Geometry check sheet. Reference: the model listing, model coordinates, mm. Face numbers are marked on the shaded views. A direction names the side the tool comes from. Round coordinates to 2 decimals unless told otherwise and drop trailing zeros. Loops run counter-clockwise (first coordinate to the right, second up) from the corner with the lowest first, then second, coordinate; pieces in that order, holes last. Notation, with made-up numbers: M 50,52 L 56,52 A20 cw 56,87 Z; hole C -35.75,31 d8. An arc over 180 degrees is marked long. Answer in a Markdown table with one row per item. Add a question column.
```python
from build123d import *

# Parameters (mm, degrees)
SKETCH1_W             = 150
SKETCH1_H             = 300
BOSS_EXTRUDE1_DEPTH   = 40
SKETCH2_R             = 25
BOSS_EXTRUDE2_DEPTH   = 5
SKETCH3_W             = 40
SKETCH3_H             = 120
CUT_EXTRUDE1_DEPTH    = 5
CUT_EXTRUDE2_DEPTH    = 5
CHAMFER2_SIZE         = 10
CHAMFER3_SIZE         = 2
CHAMFER4_SIZE         = 1
CHAMFER5_SIZE         = 1
CHAMFER6_SIZE         = 6
BODY_MOVE_COPY1_ANGLE = 120


with BuildPart() as part:
    # Sketch1 → Boss-Extrude1 (new, symmetric)
    with BuildSketch(Plane(origin=(0, 0, 0), x_dir=(1, 0, 0), z_dir=(0, 1, 0))):
        Rectangle(SKETCH1_W, SKETCH1_H)
    extrude(amount=BOSS_EXTRUDE1_DEPTH, both=True)

    # Sketch2 → Boss-Extrude2 (add)
    with BuildSketch(Plane.XY.offset(150)):
        with Locations(Location((-40, 0, 0), (0, 0, 180))):
            Circle(SKETCH2_R)
        with Locations(Location((40, 0, 0), (0, 0, 180))):
            Circle(SKETCH2_R)
    boss_extrude2 = extrude(amount=BOSS_EXTRUDE2_DEPTH)

    # Sketch3 → Cut-Extrude1 (cut)
    with BuildSketch(Plane(origin=(0, 40, 0), x_dir=(1, 0, 0), z_dir=(0, 1, 0))):
        Rectangle(SKETCH3_W, SKETCH3_H)
    extrude(amount=-CUT_EXTRUDE1_DEPTH, mode=Mode.SUBTRACT)

    # Sketch4 → Cut-Extrude2 (cut)
    with BuildSketch(Plane(origin=(0, 40, 0), x_dir=(1, 0, 0), z_dir=(0, 1, 0))):
        Polygon((0, -130), (-45, -90), (-26.937608132, -90), (0, -113.944540562), (26.937608132, -90), (45, -90), align=None)
    extrude(amount=-CUT_EXTRUDE2_DEPTH, mode=Mode.SUBTRACT)

    # Chamfer2
    chamfer2_edges = [part.edges().sort_by_distance(p)[0] for p in [
        (75, 40, 0),
        (-75, 40, 0),
        (75, -40, 0),
        (-75, -40, 0),
    ]]
    chamfer(chamfer2_edges, length=CHAMFER2_SIZE)

    # Chamfer3
    chamfer3_edges = [part.edges().sort_by_distance(p)[0] for p in [
        (-20, 35, 0),
        (0, 35, -60),
        (20, 35, 0),
        (0, 35, 60),
        (-20, 40, 0),
        (0, 40, 60),
        (20, 40, 0),
        (0, 40, -60),
        (22.5, 35, 110),
        (-22.5, 35, 110),
        (-35.968804066, 35, 90),
        (-13.468804066, 35, 101.972270281),
        (13.468804066, 35, 101.972270281),
        (35.968804066, 35, 90),
        (22.5, 40, 110),
        (35.968804066, 40, 90),
        (13.468804066, 40, 101.972270281),
        (-13.468804066, 40, 101.972270281),
        (-35.968804066, 40, 90),
        (-22.5, 40, 110),
    ]]
    chamfer(chamfer3_edges, length=CHAMFER3_SIZE)

    # Mirror1: Boss-Extrude2 across plane
    add(boss_extrude2.mirror(Plane.XY))

    # Chamfer4
    chamfer4_edges = [part.edges().sort_by_distance(p)[0] for p in [
        (-15, 0, -155),
        (65, 0, -155),
        (-15, 0, 155),
        (65, 0, 155),
    ]]
    chamfer(chamfer4_edges, length=CHAMFER4_SIZE)

    # Chamfer5
    chamfer5_edges = [part.edges().sort_by_distance(p)[0] for p in [
        (-15, 0, 150),
        (-15, 0, -150),
        (65, 0, -150),
        (65, 0, 150),
    ]]
    chamfer(chamfer5_edges, length=CHAMFER5_SIZE)

    # Chamfer6
    chamfer6_edges = [part.edges().sort_by_distance(p)[0] for p in [
        (75, 0, -150),
        (75, 0, 150),
        (0, -40, -150),
        (-75, 0, -150),
        (0, 40, -150),
        (-70, 35, -150),
        (70, 35, -150),
        (-70, -35, -150),
        (70, -35, -150),
        (0, -40, 150),
        (0, 40, 150),
        (-75, 0, 150),
        (-70, 35, 150),
        (70, 35, 150),
        (-70, -35, 150),
        (70, -35, 150),
    ]]
    chamfer(chamfer6_edges, length=CHAMFER6_SIZE)


with BuildPart() as part_1:
    # Body-Move/Copy1: moved
    add(part.part.rotate(Axis((0, 0, 0), (0.5773502691896252, 0.5773502691896252, 0.5773502691896272)), BODY_MOVE_COPY1_ANGLE))


solid = part_1.part
```
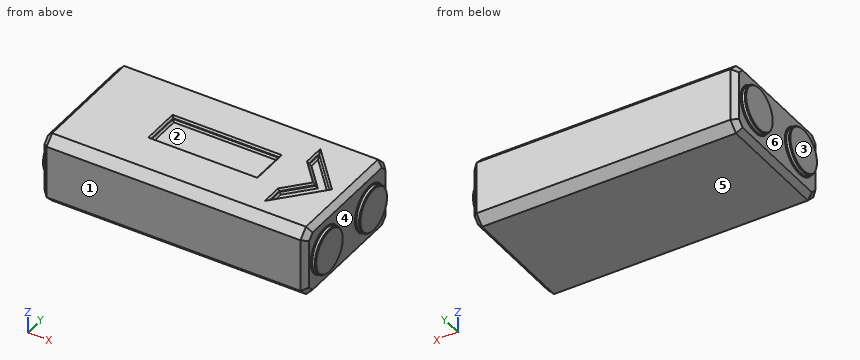
1) Set-up check for the marked faces 5 and 6: record each of +Z, -Z, +X, -X, +Y, -Y from which the full face is reachable in a straight line by a thin tool's end or side.
2) Go/stop test with flat-tipped pins: pin 1 (0.8 mm diameter, centred on y = 9, z = 37.5, fed in from -X); pin 2 (0.5 mm diameter, centred on x = 26, z = 37.5, fed in from +Y); pin 3 (1.1 mm diameter, centred on y = 34, z = 37.5, fed in from +X). Record where each tip stops, or that it passes through.
3) Cross-section at B-B, the plane y = 3. Record the boundary of the cut face in (x, z).
4) Draft check along X on the marked faces 1, 2, 3 and 4. Enter one of: +X half, -X half, draft (parallel to the pull), parting line (faces both ways), or undercut.
5) Thickness scan on L1, parallel to X at y = 66.5, z = 0; L2, parallel to Z at x = -18.5, y = -11; L3, parallel to Y at x = 18, z = 37.5. Record the ranges inside material, lowest first. Write a range as [from, to].
6) Cross-section at A-A, the plane x = -13.5. Record the boundary of the cut face in (y, z).
7) Cross-section at C-C, the plane x = 76. Record the boundary of the cut face in (y, z).
Worked answers:
| question | item | result |
|---|---|---|
| 1 | face 5 | -Z, +X, -X, +Y, -Y |
| 1 | face 6 | -X |
| 2 | pin 1 | stops at x = -146.9 |
| 2 | pin 2 | stops at y = 67.75 |
| 2 | pin 3 | stops at x = 147.05 |
| 3 | outline | M -150,-34 L -144,-40 L 144,-40 L 150,-34 L 150,34 L 144,40 L 130.01,40 L 127.33,38 L 127.33,37 L 124.66,35 L 113.95,35 L 111.28,37 L 111.28,38 L 108.6,40 L 62,40 L 60,38 L 60,37 L 58,35 L -58,35 L -60,37 L -60,38 L -62,40 L -144,40 L -150,34 Z |
| 4 | face 1 | draft |
| 4 | face 2 | undercut |
| 4 | face 3 | -X half |
| 4 | face 4 | +X half |
| 5 | L1 | x = [-150, 150] |
| 5 | L2 | z = [-40, 35] |
| 5 | L3 | y = [-67.5, -20], [20, 67.5] |
| 6 | outline | M -75,-30 L -65,-40 L 65,-40 L 75,-30 L 75,30 L 65,40 L 22,40 L 20,38 L 20,37 L 18,35 L -18,35 L -20,37 L -20,38 L -22,40 L -65,40 L -75,30 Z |
| 7 | outline | M -75,-30 L -65,-40 L 65,-40 L 75,-30 L 75,30 L 65,40 L -65,40 L -75,30 Z |
